Work out the finished part from the listing and answer in its coordinate system (mm). A direction names the side the tool comes from. Round coordinates to 2 decimals unless told otherwise and drop trailing zeros. Write each loop counter-clockwise with the first axis right and the second up, starting at its lowest first coordinate (ties: lowest second). Pieces come first, ordered by that corner, then holes. Notation, with made-up numbers: M -19.5,43.5 L 35.5,43.5 A22 ccw 35.5,55.5 Z; hole C 52,69 d11. An arc over 180 degrees is marked long. Answer in a Markdown table with one row per item.
```python
from build123d import *

# Parameters (mm, degrees)
CHAMFER_1_SIZE                       = 1
CHAMFER_2_SIZE                       = 1
FILLET_1_R                           = 0.2
SKETCH_5_R                           = 1.2
CUT_EXTRUDE_2_DEPTH                  = 2
CHAMFER_3_SIZE                       = 0.5
PATTERN_CIRCULAR_1_COUNT             = 2
CHAMFER_3_OF_PATTERN_CIRCULAR_1_SIZE = 0.5


with BuildPart() as part:
    # 스케치3 → 회전2 (revolve)
    with BuildSketch(Plane(origin=(0, 0, 0), x_dir=(1, 0, 0), z_dir=(0, 1, 0)), mode=Mode.PRIVATE) as revolve_2_sk:
        Polygon((11.1, 0), (11.1, -2.4), (8.6, -2.4), (8.6, -4.2), (11.1, -6.2), (11.1, -8.2), (9.5, -8.2), (9.5, -11.2), (9.85, -11.55), (9.85, -16.45), (9.5, -16.8), (9.5, -19.8), (3.25, -19.8), (3.25, -11.8), (4.4, -11.8), (4.4, -10), (3.4, -10), (3.4, -8.5), (6.1, -7.77653718), (6.1, 0), align=None)
    revolve(revolve_2_sk.sketch.rotate(Axis((0, 0, 0), (0, 0, 1)), 180), axis=Axis((0, 0, 0), (0, 0, 1)))

    # 모따기1
    chamfer_1_edges = [part.edges().sort_by_distance(p)[0] for p in [
        (9.5, 0, 19.8),
        (6.1, 0, 0),
    ]]
    chamfer(chamfer_1_edges, length=CHAMFER_1_SIZE)

    # 모따기2
    chamfer_2_edges = [part.edges().sort_by_distance(p)[0] for p in [
        (11.1, 0, 0),
    ]]
    chamfer(chamfer_2_edges, length=CHAMFER_2_SIZE)

    # 필렛1
    fillet_1_edges = [part.edges().sort_by_distance(p)[0] for p in [
        (11.1, 0, 2.4),
    ]]
    fillet(fillet_1_edges, radius=FILLET_1_R)

    # 스케치5 → 컷-돌출2 (cut)
    with BuildSketch(Plane(origin=(0, 11.1, 0), x_dir=(1, 0, 0), z_dir=(0, 1, 0))):
        with Locations(Location((0, -14, 0), (0, 0, 270))):
            Circle(SKETCH_5_R)
    cut_extrude_2 = extrude(amount=-CUT_EXTRUDE_2_DEPTH, mode=Mode.SUBTRACT)

    # 모따기3
    chamfer_3_edges = [part.edges().sort_by_distance(p)[0] for p in [
        (0, 9.1, 12.8),
    ]]
    chamfer(chamfer_3_edges, length=CHAMFER_3_SIZE)

    # 원형 패턴1: 컷-돌출2 ×2 about axis
    pattern_circular_1_axis = Axis((0, 0, 0), (0, 0, -1))
    for i in range(1, PATTERN_CIRCULAR_1_COUNT):
        add(cut_extrude_2.rotate(pattern_circular_1_axis, i * 360 / PATTERN_CIRCULAR_1_COUNT), mode=Mode.SUBTRACT)

    # 모따기3 of 원형 패턴1
    chamfer_3_of_pattern_circular_1_edges = [part.edges().sort_by_distance(p)[0] for p in [
        (0, -9.1, 12.8),
    ]]
    chamfer(chamfer_3_of_pattern_circular_1_edges, length=CHAMFER_3_OF_PATTERN_CIRCULAR_1_SIZE)


solid = part.part
```
1. The part is cut by section C-C (z = 14). Determine the outline of the cut face in (x, y), plus the area to 3 significant figures.
Calculated:
| item | result |
|---|---|
| outline | M -1.2,-9.78 L -1.2,-9.6 L -0.7,-9.1 L 0.7,-9.1 L 1.2,-9.6 L 1.2,-9.78 A9.85 ccw 1.2,9.78 L 1.2,9.6 L 0.7,9.1 L -0.7,9.1 L -1.2,9.6 L -1.2,9.78 A9.85 ccw Z; hole C 0,0 d6.5 |
| area | 269 mm² |
2. A tool of negligible diameter and unlimited length cuts with its end or side. For faces 5 (the cylindrical face through (1.445, -11.006, 7.214)), 6 (the cylindrical face through (0.74, 3.32, 9.24)), 7 (the flat face through (-2, 3, 11.8)), 8 (the cylindrical face through (2.059, 9.274, 17.814)), from which of +Z, -Z, +X, -X, +Y, -Y can it reach the whole face along a straight path? Write none if from no direction.
Calculated:
| item | result |
|---|---|
| face 5 | +Z, -Z |
| face 6 | -Z |
| face 7 | none |
| face 8 | +Z |
3. Given pin 1 (4.5 mm diameter, centred on x = 1, y = 1.5, fed in from -Z); pin 2 (1.5 mm diameter, centred on x = 1, z = 4.5, fed in from +Y); pin 3 (1.5 mm diameter, centred on x = 0, z = 14, fed in from -Y); pin 4 (6 mm diameter, centred on x = 0, y = 0, fed in from +Z), each flat-ended and moving along its own axis, determine where each tip first touches the part or whether it passes through.
Calculated:
| item | result |
|---|---|
| pin 1 | stops at z = 8.33 |
| pin 2 | stops at y = 9.86 |
| pin 3 | stops at y = -9.15 |
| pin 4 | passes through |
4. The part is cut by section B-B (z = 17.5). Determine the outline of the cut face in (x, y), plus the area to 3 significant figures.
Calculated:
| item | result |
|---|---|
| outline | C 0,0 d19; hole C 0,0 d6.5 |
| area | 250 mm² |
5. Consider line 1 along Y through (x, z) = (0, 8.9); line 2 along Z through (x, y) = (0, 9.75); line 3 along Y through (x, z) = (-1, 14.5). Determine where each line is inside the solid, lowest interval first. Write a range as from..to.
Calculated:
| item | result |
|---|---|
| line 1 | y = -9.5..-3.4, 3.4..9.5 |
| line 2 | z = 0..2.4, 5.12..8.2, 11.45..12.8, 15.2..16.55 |
| line 3 | y = -9.52..-3.09, 3.09..9.52 |
6. The part is cut by section A-A (z = 3.5). Determine the outline of the cut face in (x, y).
Calculated:
| item | result |
|---|---|
| outline | C 0,0 d17.2; hole C 0,0 d12.2 |
7. Determine the mould class of faces 1 (the cylindrical face through (2.579, 1.978, 15.744)), 2 (the flat face through (0, -9.1, 14)), 3 (the cylindrical face through (8.59, -0.38, 3.31)), 4 (the flat face through (-2, 3, 10)) for opening direction Y: released by +Y, released by -Y, zero draft, split by the parting line, or undercut.
Calculated:
| item | result |
|---|---|
| face 1 | undercut |
| face 2 | released by -Y |
| face 3 | split by the parting line |
| face 4 | undercut |
